from build123d import *

# Parameters (mm, degrees)
F0_W     = 101.6
F0_H     = 203.2
F0_R     = 21.411557
F1_DEPTH = 25.4


with BuildPart() as f1:
    # F0 (on Front) → F1 (new body)
    with BuildSketch(Plane.XZ):
        with Locations((-45.625693, 4.884522)):
            Rectangle(F0_W, F0_H)
        with Locations((-45.625693, 30.284522)):
            Circle(F0_R, mode=Mode.SUBTRACT)
        Polygon((-45.625693, 157.284522), (-96.425693, 106.484522), (5.174307, 106.484522), align=None)
    extrude(amount=F1_DEPTH)


solid = f1.part
Geometry check sheet. Reference: the model listing, model coordinates, mm. Coordinates: 2 decimals unless noted, no trailing zeros. Write each loop counter-clockwise with the first axis right and the second up, starting at its lowest first coordinate (ties: lowest second). Pieces come first, ordered by that corner, then holes. Notation, with made-up numbers: (-30.5, 49.5) -> (-4.5, 49.5) arc R16 cw to (-4.5, 80.5) -> close; hole circle Ø9 at (-21.75, 38). An arc over 180 degrees is marked (long way). One line per question, with ' | ' between items.
1. Thickness scan on probe 1 along X at (y, z) = (-14.75, 30); probe 2 along Z at (x, y) = (-48, -14); probe 3 along X at (y, z) = (-7, 11). Record the ranges inside material, lowest first. Write a range as from..to.
Answers:
probe 1: x = -96.43..-67.04, -24.22..5.17 | probe 2: z = -96.72..9.01, 51.56..154.91 | probe 3: x = -96.43..-54.93, -36.32..5.17
2. Depth check by flat-ended pin: pin 1 Ø4 at (x, z) = (-40.5, -57.5) entering from +Y; pin 2 Ø5 at (x, y) = (-20.5, -13) entering from +Z; pin 3 Ø8 at (y, z) = (-12.5, 116) entering from -X; pin 4 Ø5 at (x, y) = (-34.5, -12) entering from +Z. Enter the tip coordinate at first touch or a pass-through.
Answers:
pin 1: stops at y = 0 | pin 2: stops at z = 134.66 | pin 3: stops at x = -90.91 | pin 4: stops at z = 148.66
3. Cross-section at C-C on z = 129. Record the cut outline in (x, y).
Answers:
outline: (-73.91, -25.4) -> (-17.34, -25.4) -> (-17.34, 0) -> (-73.91, 0) -> close
4. Cross-section at A-A on x = -34.5. Record the cut outline in (y, z), and give its area (3 significant figures).
Answers:
outline: (-25.4, -96.72) -> (0, -96.72) -> (0, 11.99) -> (-25.4, 11.99) -> close; (-25.4, 48.58) -> (0, 48.58) -> (0, 146.16) -> (-25.4, 146.16) -> close | area: 5,240 mm²
5. Cross-section at D-D on x = -51. Record the cut outline in (y, z).
Answers:
outline: (-25.4, -96.72) -> (0, -96.72) -> (0, 9.56) -> (-25.4, 9.56) -> close; (-25.4, 51.01) -> (0, 51.01) -> (0, 151.91) -> (-25.4, 151.91) -> close
6. Cross-section at B-B on y = -3.75. Record the cut outline in (x, z), and give its area (3 significant figures).
Answers:
outline: (-96.43, -96.72) -> (5.17, -96.72) -> (5.17, 106.48) -> (-45.63, 157.28) -> (-96.43, 106.48) -> close; hole circle Ø42.82 at (-45.63, 30.28) | area: 21,800 mm²
7. Draft check along Z on faces 1 (the flat face through (-70.67, -12.52, 132.24)), 2 (the flat face through (-46, 0, 4)), 3 (the cylindrical face through (-67.017, -12.522, 31.226)), 4 (the flat face through (-46, -13, -96.715)). Enter one of: +Z half, -Z half, draft (parallel to the pull), parting line (faces both ways), or undercut.
Answers:
face 1: +Z half | face 2: draft | face 3: undercut | face 4: -Z half
